from build123d import *

# Parameters (mm, degrees)
BOSS_EXTRUDE1_DEPTH   = 12.7
BOSS_EXTRUDE1_2_DEPTH = 12.7
BOSS_EXTRUDE2_DEPTH   = 12.7
BOSS_EXTRUDE3_DEPTH   = 6.35
SKETCH4_R             = 1.5875
CUT_EXTRUDE1_DEPTH    = 20.32
SKETCH5_W             = 7.9375
SKETCH5_H             = 3.175
CUT_EXTRUDE2_DEPTH    = 12.7


with BuildPart() as part:
    # Sketch1 → Boss-Extrude1 (new body)
    with BuildSketch(Plane(origin=(0, 0, 0), x_dir=(0, 0, -1), z_dir=(1, 0, 0))):
        Polygon((34.925, 15.875), (34.925, 12.7), (3.175, 12.7), (3.175, 13.6525), (0, 13.6525), (-3.175, 13.6525), (-3.175, 12.7), (-34.925, 12.7), (-34.925, 15.875), align=None)
    extrude(amount=BOSS_EXTRUDE1_DEPTH)



with BuildPart() as body_2:
    # Sketch1 → Boss-Extrude1 2 (new body)
    with BuildSketch(Plane(origin=(0, 0, 0), x_dir=(0, 0, -1), z_dir=(1, 0, 0))):
        Polygon((-34.925, -15.875), (-34.925, -12.7), (-3.175, -12.7), (-3.175, -13.6525), (0, -13.6525), (3.175, -13.6525), (3.175, -12.7), (34.925, -12.7), (34.925, -15.875), align=None)
    extrude(amount=BOSS_EXTRUDE1_2_DEPTH)


with BuildPart() as part_1:
    add(part.part)

    add(body_2.part)  # Boss-Extrude2 merges body 2
    # Sketch1_3 → Boss-Extrude2 (add)
    with BuildSketch(Plane(origin=(0, 0, 0), x_dir=(0, 0, -1), z_dir=(1, 0, 0))):
        Polygon((34.925, 15.875), (34.925, 12.7), (3.175, 12.7), (3.175, 13.6525), (0, 13.6525), (-3.175, 13.6525), (-3.175, 12.7), (-34.925, 12.7), (-34.925, 15.875), align=None)
        Polygon((34.925, -12.7), (34.925, 12.7), (3.175, 12.7), (3.175, 13.6525), (0, 13.6525), (-3.175, 13.6525), (-3.175, 12.7), (-34.925, 12.7), (-34.925, -12.7), (-3.175, -12.7), (-3.175, -13.6525), (0, -13.6525), (3.175, -13.6525), (3.175, -12.7), align=None)
        Polygon((-34.925, -15.875), (-34.925, -12.7), (-3.175, -12.7), (-3.175, -13.6525), (0, -13.6525), (3.175, -13.6525), (3.175, -12.7), (34.925, -12.7), (34.925, -15.875), align=None)
    extrude(amount=-BOSS_EXTRUDE2_DEPTH)

    # Sketch3 → Boss-Extrude3 (add)
    with BuildSketch(Plane(origin=(0, 0, -34.925), x_dir=(-1, 0, 0), z_dir=(0, 0, -1))):
        with BuildLine():
            Line((-39.189487758, -22.225), (12.7, -22.225))
            Line((12.7, -22.225), (12.7, -15.875))
            Line((12.7, -15.875), (-12.7, -15.875))
            Line((-12.7, -15.875), (-12.7, -12.7))
            Line((-12.7, -12.7), (0, -12.7))
            Line((0, -12.7), (0, 12.7))
            Line((0, 12.7), (-12.7, 12.7))
            Line((-12.7, 12.7), (-12.7, 15.875))
            Line((-12.7, 15.875), (12.7, 15.875))
            Line((12.7, 15.875), (12.7, 22.225))
            Line((12.7, 22.225), (-39.189487758, 22.225))
            ThreePointArc((-39.189487758, 22.225), (-31.364807909, 12.314807909), (-28.575, 0))
            ThreePointArc((-28.575, 0), (-31.364807909, -12.314807909), (-39.189487758, -22.225))
        make_face()
        Polygon((-12.7, 15.875), (-12.7, 12.7), (0, 12.7), (0, -12.7), (-12.7, -12.7), (-12.7, -15.875), (12.7, -15.875), (12.7, 15.875), align=None)
    boss_extrude3 = extrude(amount=BOSS_EXTRUDE3_DEPTH)

    # Mirror1: Boss-Extrude3 across plane
    add(boss_extrude3.mirror(Plane.XY))

    # Sketch4 → Cut-Extrude1 (cut)
    with BuildSketch(Plane(origin=(0, 15.875, 0), x_dir=(1, 0, 0), z_dir=(0, 1, 0))):
        with Locations((-6.35, 22.225)):
            Circle(SKETCH4_R)
        with Locations((-6.35, -22.225)):
            Circle(SKETCH4_R)
    extrude(amount=-CUT_EXTRUDE1_DEPTH, mode=Mode.SUBTRACT)

    # Sketch5 → Cut-Extrude2 (cut)
    with BuildSketch(Plane.ZY.offset(12.7)):
        with Locations((-22.225, 4.7625)):
            Rectangle(SKETCH5_W, SKETCH5_H)
        with Locations((22.225, 4.7625)):
            Rectangle(SKETCH5_W, SKETCH5_H)
    extrude(amount=-CUT_EXTRUDE2_DEPTH, mode=Mode.SUBTRACT)


solid = part_1.part
Read the model definition and answer for the solid it produces. Units are mm, in the model's axes. A direction names the side the tool comes from. Give positions to 0.01 mm unless a question says otherwise; leave off trailing zeros. Write each loop counter-clockwise with the first axis right and the second up, starting at its lowest first coordinate (ties: lowest second). Pieces come first, ordered by that corner, then holes. Notation, with made-up numbers: (65.5, 30) - (89.5, 30) arc R23 ccw to (89.5, 68) - close; hole circle Ø2 at (67.5, 43). An arc over 180 degrees is marked (long way). Answer in a Markdown table with one row per item. Add a question column.
Item 1: Section C-C, the plane y = 17 is taken. Write down the section's boundary in (x, z) (3 decimals), and give its area (3 significant figures).
Item 2: Section D-D, the plane z = -34 is taken. Write down the section's boundary in (x, y) (3 decimals).
Item 3: Determine the mould class of faces 6 (the face through (-5.497, 11.179, -23.564)), 7 (the face through (6, 12.7, -19)), 8 (the face through (12.7, 14, 0)) for opening direction X: pulls with the +X half, pulls with the -X half, needs draft (parallel to the pull), parting line crosses it, or undercut.
Item 4: Find the intervals of material crossed by L1, parallel to Z at x = -6.35, y = 14 (1 decimal); L2, parallel to Z at x = -3.5, y = 5.5 (3 decimals); L3, parallel to Z at x = 20, y = -6 (3 decimals), in increasing order.
Item 5: Section A-A, the plane x = 25.5 is taken. Write down the section's boundary in (y, z) (3 decimals).
Item 6: A tool of negligible diameter and unlimited length cuts with its end or side. For faces 1 (the face through (-6, 5, -26.194)), 2 (the face through (-5.497, -0.582, -23.564)), 3 (the face through (0, -15.875, 0)), 4 (the face through (0, 15.875, 0)), 5 (the face through (6, 13.652, 0)), from which of +Z, -Z, +X, -X, +Y, -Y can it reach the whole face along a straight path? Write none if from no direction.
Item 7: Section B-B, the plane x = 6.5 is taken. Write down the section's boundary in (y, z) (1 decimal).
Item 8: Flat-ended cylindrical pins translate along their axes: P1, Ø5, axis at x = -6.35, z = 22.225, coming from the -Y side (3 decimals); P2, Ø3.5, axis at x = -6, z = -22, coming from the +Y side (3 decimals); P3, Ø3, axis at x = 33.5, y = -13.5, coming from the -Z side (3 decimals); P4, Ø1.6, axis at y = -14.5, z = 12, coming from the +X side. Find the tip coordinate at first contact, or state that the pin passes through.
Recorded:
| question | item | result |
|---|---|---|
| 1 | outline | (-12.7, -41.275) - (34.182, -41.275) - (34.182, -34.925) - (-12.7, -34.925) - close; (-12.7, 34.925) - (34.182, 34.925) - (34.182, 41.275) - (-12.7, 41.275) - close |
| 1 | area | 595 mm2 |
| 2 | outline | (-12.7, -15.875) - (12.7, -15.875) - (12.7, -12.7) - (0, -12.7) - (0, 12.7) - (12.7, 12.7) - (12.7, 15.875) - (-12.7, 15.875) - close |
| 3 | face 6 | undercut |
| 3 | face 7 | needs draft |
| 3 | face 8 | pulls with the +X half |
| 4 | L1 | z = -41.3 to -23.8, -20.6 to 20.6, 23.8 to 41.3 |
| 4 | L2 | z = -41.275 to -26.194, -18.256 to 18.256, 26.194 to 41.275 |
| 4 | L3 | z = -41.275 to -34.925, 34.925 to 41.275 |
| 5 | outline | (-22.225, -41.275) - (22.225, -41.275) - (22.225, -34.925) - (-22.225, -34.925) - close; (-22.225, 34.925) - (22.225, 34.925) - (22.225, 41.275) - (-22.225, 41.275) - close |
| 6 | face 1 | +X, -X |
| 6 | face 2 | +Y |
| 6 | face 3 | +X, -X, -Y |
| 6 | face 4 | +X, -X, +Y |
| 6 | face 5 | +X |
| 7 | outline | (-22.2, -41.3) - (22.2, -41.3) - (22.2, -34.9) - (15.9, -34.9) - (15.9, 34.9) - (22.2, 34.9) - (22.2, 41.3) - (-22.2, 41.3) - (-22.2, 34.9) - (-15.9, 34.9) - (-15.9, -34.9) - (-22.2, -34.9) - close; hole (-13.7, -3.2) - (-12.7, -3.2) - (-12.7, -34.9) - (12.7, -34.9) - (12.7, -3.2) - (13.7, -3.2) - (13.7, 3.2) - (12.7, 3.2) - (12.7, 34.9) - (-12.7, 34.9) - (-12.7, 3.2) - (-13.7, 3.2) - close |
| 8 | P1 | stops at y = -15.875 |
| 8 | P2 | stops at y = 15.875 |
| 8 | P3 | stops at z = -41.275 |
| 8 | P4 | stops at x = 12.7 |
